The listing builds one solid part. Answer for the finished solid, in the listing's coordinates (mm). A direction names the side the tool comes from. Coordinates: 2 decimals unless noted, no trailing zeros. Order: outer loops, then holes, each group sorted by start corner. A loop starts at its lowest first (then second) coordinate and runs counter-clockwise, first axis right, second up. Notation, with made-up numbers: (74.25, 71) -> (128.25, 71) arc R19 ccw to (128.25, 78) -> close; hole circle Ø4 at (-29, 63.25). An arc over 180 degrees is marked (long way). Answer in a Markdown table with one row per item.
Autodesk Fusion 360 part; units mm, degrees
sketch "Sketch1" plane through (0, 0, 0) normal (0, 1, 0) x (1, 0, 0)
  circle A0 centre (0, 0) radius 4
  circle A1 centre (0, 0) radius 7.5
  circle A2 centre (0, 0) radius 20
  circle A3 centre (0, 0) radius 15 construction
  circle A4 centre (0, -15) radius 2
  circle A5 centre (15, 0) radius 2
  circle A6 centre (0, 15) radius 2
  circle A7 centre (-15, 0) radius 2
  dimension "d1" = 8
  dimension "d2" = 15
  dimension "d3" = 40
  dimension "d4" = 4
  dimension "d6" = 360
extrude "Extrude1" add sketch "Sketch1" along normal blind 15 contours A1
extrude "Extrude2" add sketch "Sketch1" against normal blind 4 contours A1 | A2
fillet "Fillet1" radius 0.5 2 edges at (-18.6465, -4, -7.2323) (-18.6465, 0, 7.2323)
fillet "Fillet2" radius 1 2 edges at (-6.9925, 0, 2.7121) (-6.9925, 15, 2.7121)
hole "Hole1" at (0, 7.8114, 7.5) direction (0, 0, -1) diameter 3.332 depth 8 tip angle 118
(1) For a pull along X with two mould halves and no side action, classify faces 1 (the cylindrical face through (-1.63, 7.41, -7.32)), 2 (the flat face through (3, 15, -3)), 3 (the cylindrical face through (0, -2, 13)), 4 (the cylindrical face through (-16.6, -2, 1.2)) as released by +X, released by -X, zero draft, split by the parting line, or undercut.
Check values:
| item | result |
|---|---|
| face 1 | split by the parting line |
| face 2 | zero draft |
| face 3 | undercut |
| face 4 | undercut |
(2) A cutting plane is placed at C-C, the plane y = 13.25. Determine the outline of the cut face in (x, z), then the cut area to 3 significant figures.
Check values:
| item | result |
|---|---|
| outline | circle Ø15 at (0, 0); hole circle Ø8 at (0, 0) |
| area | 126 mm² |
(3) Which of the six approach directions +Z, -Z, +X, -X, +Y, -Y give full straight-line access (tool end or side, diameter ignored) to faces 5 (the cylindrical face through (1.846, 5.367, -3.549)), 6 (the cylindrical face through (0.638, 6.272, 5.541)), 7 (the flat face through (8, 0, 4))?
Check values:
| item | result |
|---|---|
| face 5 | +Y, -Y |
| face 6 | +Z |
| face 7 | +Y |
(4) Find the intervals of material crossed by line 1 along X through (y, z) = (-2.95, 0); line 2 along Z through (x, y) = (0, 4.25), in increasing order. Write a range as from..to.
Check values:
| item | result |
|---|---|
| line 1 | -20..-17, -13..-4, 4..13, 17..20 |
| line 2 | -7.5..-4, 4..7.5 |
(5) A cutting plane is placed at D-D, the plane y = 8.75. Determine the outline of the cut face in (x, z).
Check values:
| item | result |
|---|---|
| outline | (-1.38, 3.76) -> (-1.38, 7.37) arc R7.5 ccw (long way) to (1.38, 7.37) -> (1.38, 3.76) arc R4 cw (long way) to start |
(6) Flat-ended cylindrical pins translate along their axes: pin 1 (3 mm diameter, centred on x = 0, z = -15, fed in from +Y); pin 2 (3 mm diameter, centred on x = -7.5, y = 3.5, fed in from +Z); pin 3 (3 mm diameter, centred on x = 0, y = 7.81, fed in from +Z); pin 4 (1.5 mm diameter, centred on y = 5.5, z = -4, fed in from +X). Find the tip coordinate at first contact, or state that the pin passes through.
Check values:
| item | result |
|---|---|
| pin 1 | through |
| pin 2 | z = 4.5 |
| pin 3 | z = -3.71 |
| pin 4 | x = 6.76 |
(7) A cutting plane is placed at B-B, the plane x = 0. Count the separate pieces of the cut face and the enclosed holes in it, then the cut area to 3 significant figures.
Check values:
| item | result |
|---|---|
| separate pieces | 5 |
| enclosed holes | 0 |
| area | 189 mm² |
(8) A cutting plane is placed at A-A, the plane z = 0. Determine the outline of the cut face in (x, y), then the cut area to 3 significant figures.
Check values:
| item | result |
|---|---|
| outline | (-20, -3.5) arc R0.5 ccw to (-19.5, -4) -> (-17, -4) -> (-17, 0) -> (-19.5, 0) arc R0.5 ccw to (-20, -0.5) -> close; (-13, -4) -> (-4, -4) -> (-4, 15) -> (-6.5, 15) arc R1 ccw to (-7.5, 14) -> (-7.5, 1) arc R1 cw to (-8.5, 0) -> (-13, 0) -> close; (4, -4) -> (13, -4) -> (13, 0) -> (8.5, 0) arc R1 cw to (7.5, 1) -> (7.5, 14) arc R1 ccw to (6.5, 15) -> (4, 15) -> close; (17, -4) -> (19.5, -4) arc R0.5 ccw to (20, -3.5) -> (20, -0.5) arc R0.5 ccw to (19.5, 0) -> (17, 0) -> close |
| area | 201 mm² |
